Verification items for the finished model (mm, model axes). Give positions to 0.01 mm unless a question says otherwise; leave off trailing zeros. Loops run counter-clockwise (first coordinate to the right, second up) from the corner with the lowest first, then second, coordinate; pieces in that order, holes last. Notation, with made-up numbers: (1, 61) - (25, 61) arc R8 cw to (25, 74) - close; hole circle Ø9 at (83, 56.25). An arc over 180 degrees is marked (long way). One line per item, written item: value. Start each with the question number.
1. Sectioned sample at A-A (y = 171). Record the cut outline in (x, z), plus the area to 3 significant figures.
2. Sectioned sample at B-B (z = 977). Record the cut outline in (x, y).
3. Gauge pin test, flat ends, axial feed: pin 1 (12.5 mm diameter, centred on x = -5, y = 120, fed in from -Z); pin 2 (20.5 mm diameter, centred on x = 4, y = 335.5, fed in from -Z). Record the tip position at first contact, or that the pin passes through.
4. Sectioned sample at D-D (y = 373). Record the cut outline in (x, z).
5. Sectioned sample at C-C (y = 79). Record the cut outline in (x, z), plus the area to 3 significant figures.
6. Scan lines: L1, parallel to Y at x = 8, z = 1716; L2, parallel to Z at x = 53.5, y = 432; L3, parallel to Y at x = 2.5, z = 842. Record each from-to range of solid material in increasing order. Write a range as [from, to].
from build123d import *

# Parameters (mm, degrees)
F1_DEPTH = 25.4
F2_W     = 25.4
F2_H     = 25.4


with BuildPart() as f1:
    # F0 (on Top) → F1 (new body)
    with BuildSketch(Plane.XY):
        Polygon((44.7061754991, 508), (-44.7061754991, 508), (-185.8172866102, 0), (185.8172866102, 0), align=None)
        Polygon((-152.4, 25.4), (-25.4, 482.6), (25.4, 482.6), (152.4, 25.4), align=None, mode=Mode.SUBTRACT)
    extrude(amount=-F1_DEPTH)

    # F4: sweep along a path in F3
    with BuildLine(Plane.YZ) as f4_path:
        Line((508, 0), (508, 1727.2))
        Line((508, 1727.2), (406.4, 1828.8))
        Line((406.4, 1828.8), (203.2, 1828.8))
        Line((203.2, 1828.8), (101.6, 1727.2))
        Line((101.6, 1727.2), (101.6, 1625.6))
    # F2 (on Top) → F4 (sweep)
    with BuildSketch(Plane.XY):
        with Locations((0, 495.3)):
            Rectangle(F2_W, F2_H)
    sweep(path=f4_path.line, transition=Transition.RIGHT)


solid = f1.part
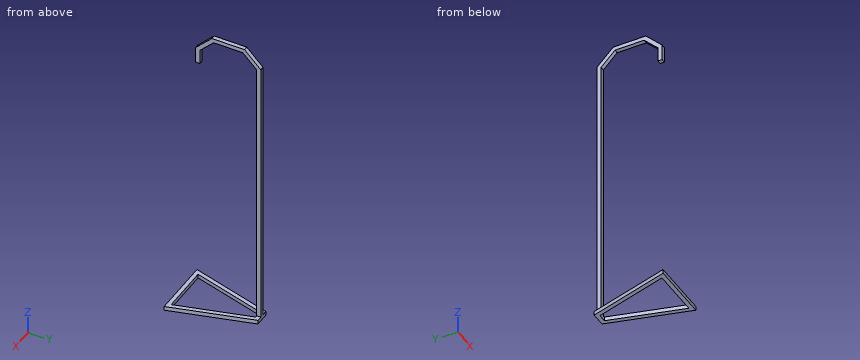
Results are:
1. outline: (-138.32, -25.4) - (-111.96, -25.4) - (-111.96, 0) - (-138.32, 0) - close; (-12.7, 1760.68) - (12.7, 1760.68) - (12.7, 1796.6) - (-12.7, 1796.6) - close; (111.96, -25.4) - (138.32, -25.4) - (138.32, 0) - (111.96, 0) - close
1. area: 2,250 mm^2
2. outline: (-12.7, 482.6) - (12.7, 482.6) - (12.7, 508) - (-12.7, 508) - close
3. pin 1: stops at z = 1625.6
3. pin 2: stops at z = 1803.4
4. outline: (-82.21, -25.4) - (-55.84, -25.4) - (-55.84, 0) - (-82.21, 0) - close; (-12.7, 1803.4) - (12.7, 1803.4) - (12.7, 1828.8) - (-12.7, 1828.8) - close; (55.84, -25.4) - (82.21, -25.4) - (82.21, 0) - (55.84, 0) - close
5. outline: (-163.87, -25.4) - (-137.51, -25.4) - (-137.51, 0) - (-163.87, 0) - close; (137.51, -25.4) - (163.87, -25.4) - (163.87, 0) - (137.51, 0) - close
5. area: 1,340 mm^2
6. L1: y = [101.6, 127], [482.6, 508]
6. L2: z = [-25.4, 0]
6. L3: y = [482.6, 508]
